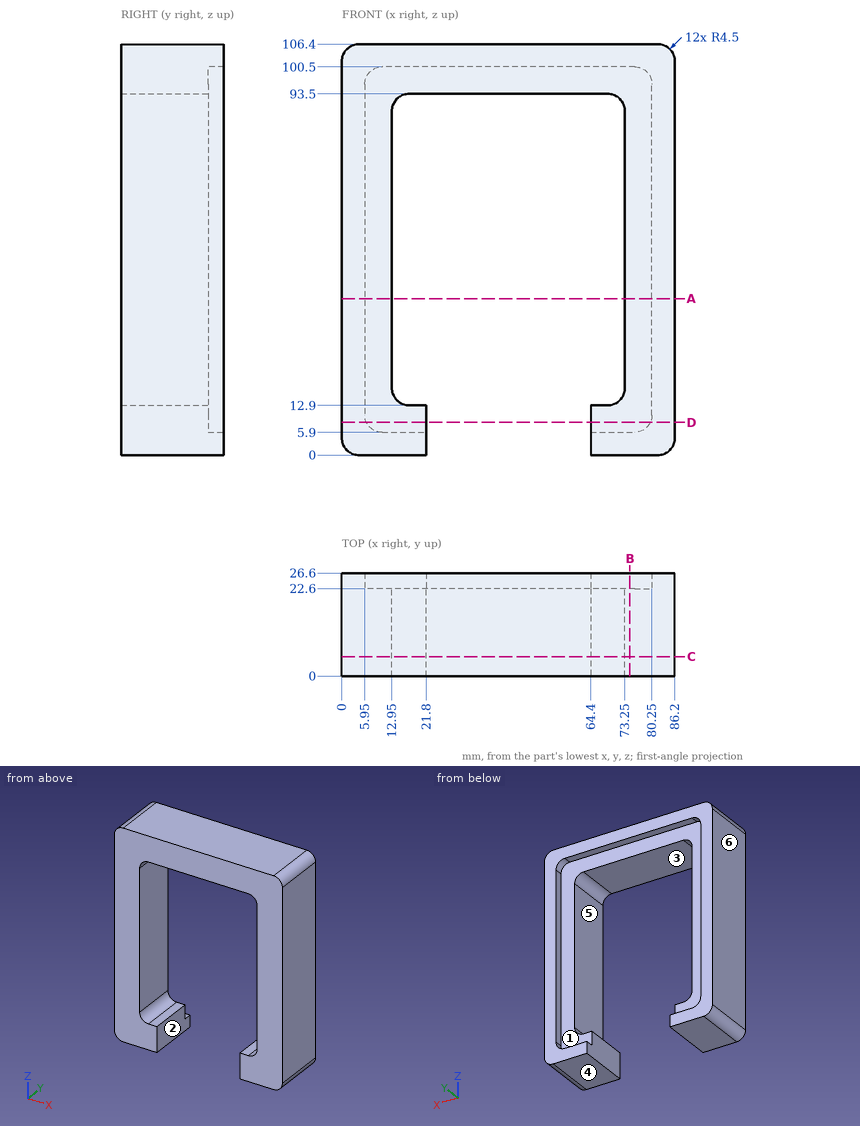
The figure shows three views and two pictorial views of one solid part (mm, origin at its lowest corner). Answer the questions. A direction names the side the tool comes from. Coordinates: 2 decimals unless noted, no trailing zeros. Write each loop counter-clockwise with the first axis right and the second up, starting at its lowest first coordinate (ties: lowest second). Pieces come first, ordered by that corner, then holes. Notation, with made-up numbers: (58.5, 57.5) -> (116.5, 57.5) arc R13 ccw to (116.5, 73.5) -> close; hole circle Ø5 at (-3.5, -33). An arc over 180 degrees is marked (long way). Return JSON: item names as keys, results as strings.
1. Determine the mould class of the marked faces 4, 5 and 6 for opening direction X: pulls with the +X half, pulls with the -X half, needs draft (parallel to the pull), parting line crosses it, or undercut.
Found:
{"face 4": "needs draft", "face 5": "undercut", "face 6": "pulls with the -X half"}
2. A cutting plane is placed at A-A (z = 40.5). Determine the outline of the cut face in (x, y), and give its area (3 significant figures).
Found:
{"outline": "(0, 0) -> (12.95, 0) -> (12.95, 22.6) -> (5.95, 22.6) -> (5.95, 26.6) -> (0, 26.6) -> close; (73.25, 0) -> (86.2, 0) -> (86.2, 26.6) -> (80.25, 26.6) -> (80.25, 22.6) -> (73.25, 22.6) -> close", "area": "633 mm2"}
3. Find the intervals of material crossed by line 1 along X through (y, z) = (2, 84.5); line 2 along X through (y, z) = (4.5, 6.5); line 3 along Z through (x, y) = (67.5, 21.25), in increasing order. Write a range as from..to.
Found:
{"line 1": "0..12.95, 73.25..86.2", "line 2": "0..21.8, 64.4..86.2", "line 3": "0..12.9, 93.5..106.4"}
4. A tool of negligible diameter and unlimited length cuts with its end or side. For the marked faces 1, 2 and 3, from which of +Z, -Z, +X, -X, +Y, -Y can it reach the whole face along a straight path? Write none if from no direction.
Found:
{"face 1": "+Y", "face 2": "-Z, +Y, -Y", "face 3": "+Y, -Y"}
5. Each of these flat-tipped pins is pushed along its axis until it touches: P1, Ø11.5, axis at x = 33, y = 12, coming from the -Z side; P2, Ø8, axis at x = 10.5, z = 94, coming from the +Y side. Where does it stop, or does it pass through?
Found:
{"P1": "z = 93.5", "P2": "y = 22.6"}
6. A cutting plane is placed at C-C (y = 5). Determine the outline of the cut face in (x, z), and give its area (3 significant figures).
Found:
{"outline": "(0, 4.5) arc R4.5 ccw to (4.5, 0) -> (21.8, 0) -> (21.8, 12.9) -> (17.45, 12.9) arc R4.5 cw to (12.95, 17.4) -> (12.95, 89) arc R4.5 cw to (17.45, 93.5) -> (68.75, 93.5) arc R4.5 cw to (73.25, 89) -> (73.25, 17.4) arc R4.5 cw to (68.75, 12.9) -> (64.4, 12.9) -> (64.4, 0) -> (81.7, 0) arc R4.5 ccw to (86.2, 4.5) -> (86.2, 101.9) arc R4.5 ccw to (81.7, 106.4) -> (4.5, 106.4) arc R4.5 ccw to (0, 101.9) -> close", "area": "3,760 mm2"}
7. A cutting plane is placed at D-D (z = 8.5). Determine the outline of the cut face in (x, y).
Found:
{"outline": "(0, 0) -> (21.8, 0) -> (21.8, 22.6) -> (6.37, 22.6) -> (6.37, 26.6) -> (0, 26.6) -> close; (64.4, 0) -> (86.2, 0) -> (86.2, 26.6) -> (79.83, 26.6) -> (79.83, 22.6) -> (64.4, 22.6) -> close"}
8. A cutting plane is placed at B-B (x = 74.5). Determine the outline of the cut face in (y, z), and give its area (3 significant figures).
Found:
{"outline": "(0, 0) -> (26.6, 0) -> (26.6, 5.9) -> (22.6, 5.9) -> (22.6, 100.5) -> (26.6, 100.5) -> (26.6, 106.4) -> (0, 106.4) -> close", "area": "2,450 mm2"}
